Build history of the part. All positions in model axes, mm. Face numbers are marked on the shaded views. A direction names the side the tool comes from. Round coordinates to 2 decimals unless told otherwise and drop trailing zeros. Write each loop counter-clockwise with the first axis right and the second up, starting at its lowest first coordinate (ties: lowest second). Pieces come first, ordered by that corner, then holes. Notation, with made-up numbers: M 3.25,11.5 L 26.25,11.5 A34 ccw 26.25,44.5 Z; hole C 49,27 d7. An arc over 180 degrees is marked long. One line per item, written item: value. Start each with the question number.
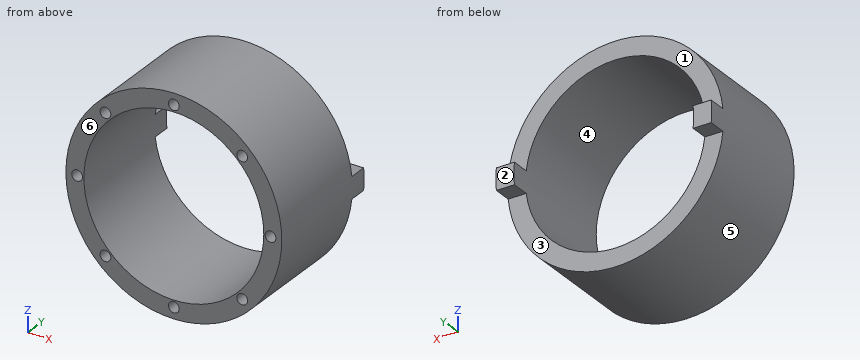
Autodesk Inventor part; units mm, degrees
ref_plane "YZ Plane" through (0, 0, 0) normal (1, 0, 0) x (0, 1, 0)
ref_plane "XZ Plane" through (0, 0, 0) normal (0, 1, 0) x (-1, 0, 0)
ref_plane "XY Plane" through (0, 0, 0) normal (0, 0, 1) x (1, 0, 0)
sketch "Sketch1" plane through (0, 0, 0) normal (0, 1, 0) x (-1, 0, 0)
  line L0 (0, 0) -> (50, 0) construction
  line L1 (0, 0) -> (50, 0) construction
  line L2 (0, 0) -> (-36, 0)
  circle A0 centre (0, 0) radius 25
  line L3 (-60, -10) -> (-60, 10)
  circle A1 centre (0, 0) radius 61
  point P0 (62.509, -33.0548)
  point P1 (12.6591, 21.558)
  point P2 (24.4148, 5.3777)
  point P3 (24.4148, -5.3777)
  point P4 (-22.9129, 10)
  point P5 (-22.9129, -10)
  point P6 (12.6591, -21.558)
  dimension "d2" = 36
  dimension "d3" = 50
  dimension "d26" = 122
extrude "Extrusion1" add sketch "Sketch1" along normal blind 5 contours A0 | A1
sketch "Sketch2" plane through (0, 5, 0) normal (0, 1, 0) x (1, 0, 0)
  circle A0 centre (0, 0) radius 20
  dimension "d6" = 40
extrude "Extrusion2" cut sketch "Sketch2" against normal up to next
sketch "Sketch3" plane through (0, 5, 0) normal (0, 1, 0) x (1, 0, 0)
  line L0 (22.1416, 4) -> (20.8701, 4)
  line L1 (22.1416, -4) -> (20.8701, -4)
  line L2 (24.6779, 4) -> (22.1416, 4)
  line L3 (24.6779, -4) -> (22.1416, -4)
  line L4 (-15.5618, -16.2506) -> (-14.5332, -15.5032)
  line L5 (-15.5618, 16.2506) -> (-14.5332, 15.5032)
  line L6 (-20.2641, -9.7784) -> (-19.2354, -9.0311)
  line L7 (-17.6137, -17.7414) -> (-15.5618, -16.2506)
  line L8 (-22.316, -11.2693) -> (-20.2641, -9.7784)
  line L9 (-20.2641, 9.7784) -> (-19.2354, 9.0311)
  line L10 (-17.6137, 17.7414) -> (-15.5618, 16.2506)
  line L11 (-22.316, 11.2693) -> (-20.2641, 9.7784)
  line L12 (-23.5374, 22.0452) -> (-13.679, 22.0452) construction
  arc A0 (-17.6137, -17.7414) -> (24.6779, -4) centre (0, 0) ccw
  arc A1 (24.6779, 4) -> (-17.6137, 17.7414) centre (0, 0) ccw
  arc A2 (-22.316, 11.2693) -> (-22.316, -11.2693) centre (0, 0) ccw
  line L13 (20.8701, 4) -> (15.8701, 4)
  line L14 (15.8701, 4) -> (15.8701, -4)
  line L15 (15.8701, -4) -> (20.8701, -4)
  line L16 (-14.5332, 15.5032) -> (-10.4881, 12.5643)
  line L17 (-10.4881, 12.5643) -> (-15.1903, 6.0922)
  line L18 (-15.1903, 6.0922) -> (-19.2354, 9.0311)
  line L19 (-19.2354, -9.0311) -> (-15.1903, -6.0922)
  line L20 (-15.1903, -6.0922) -> (-10.4881, -12.5643)
  line L21 (-10.4881, -12.5643) -> (-14.5332, -15.5032)
  circle A3 centre (-22.5, 0) radius 1.5
  circle A4 centre (0, 22.5) radius 1.5
  circle A5 centre (18.2029, 13.2252) radius 1.5
  circle A6 centre (18.2029, -13.2252) radius 1.5
  circle A7 centre (0, -22.5) radius 1.5
  circle A8 centre (0, 0) radius 4
  line L22 (0, 0) -> (8, 0)
  line L23 (8, 0) -> (8, 7.5)
  line L24 (8, 0) -> (8, -7.5)
  circle A9 centre (8, -7.5) radius 2.5
  circle A10 centre (8, 7.5) radius 2.5
  point P0 (-23.5374, -22.0452)
  point P1 (-28.2397, -15.5731)
  dimension "d9" = 36
  dimension "d10" = 5
  dimension "d11" = 5
  dimension "d12" = 3
  dimension "d13" = 3
  dimension "d14" = 3
  dimension "d15" = 3
  dimension "d16" = 3
  dimension "d17" = 8
  dimension "d18" = 8
  dimension "d19" = 7.5
  dimension "d20" = 7.5
  dimension "d21" = 5
  dimension "d22" = 5
extrude "Extrusion3" cut sketch "Sketch3" against normal up to next contours A3 | A4 | A5 | A6 | A7
sketch "Sketch5" plane through (0, 5, 0) normal (0, 1, 0) x (1, 0, 0)
  line L0 (0, 0) -> (37.5601, 0) construction
  circle A0 centre (0, 0) radius 25
  line L1 (0, 0) -> (15.7675, -27.31)
  line L2 (0, 0) -> (31.5349, 0) construction
  line L3 (0, 0) -> (19.8269, 34.3411)
  line L4 (0, 0) -> (39.6537, 0) construction
  line L5 (12.5, 21.6506) -> (15, 25.9808)
  line L6 (12.5, -21.6506) -> (15, -25.9808)
  line L7 (15, -25.9808) -> (27.9904, -18.4808)
  line L8 (27.9904, -18.4808) -> (34.9904, -30.6051)
  line L9 (34.9904, -30.6051) -> (22, -38.1051)
  line L10 (22, -38.1051) -> (15, -25.9808)
  line L11 (22, -38.1051) -> (15, -25.9808)
  line L12 (15, -25.9808) -> (2.0096, -33.4808)
  line L13 (2.0096, -33.4808) -> (9.0096, -45.6051)
  line L14 (9.0096, -45.6051) -> (22, -38.1051)
  line L15 (15, 25.9808) -> (2.0096, 33.4808)
  line L16 (2.0096, 33.4808) -> (9.0096, 45.6051)
  line L17 (9.0096, 45.6051) -> (22, 38.1051)
  line L18 (22, 38.1051) -> (15, 25.9808)
  line L19 (22, 38.1051) -> (15, 25.9808)
  line L20 (15, 25.9808) -> (27.9904, 18.4808)
  line L21 (27.9904, 18.4808) -> (34.9904, 30.6051)
  line L22 (34.9904, 30.6051) -> (22, 38.1051)
  dimension "d41" = 50
  dimension "d47" = 60
  dimension "d48" = 60
  dimension "d49" = 5
  dimension "d50" = 5
  dimension "d51" = 15
  dimension "d52" = 14
  dimension "d53" = 15
  dimension "d54" = 15
  dimension "d55" = 14
  dimension "d56" = 15
extrude "Extrusion5" cut sketch "Sketch5" against normal up to next contours L7 L8 L9 L10 L1 | L1 L10 L14 L13 L12 | L15 L16 L17 L18 L3 | L3 L18 L22 L21 L20
sketch "Sketch6" plane through (0, 0, 0) normal (0, -1, 0) x (1, 0, 0)
  circle A0 centre (0, 0) radius 25
  circle A1 centre (0, 0) radius 28.75
  circle A2 centre (0, 0) radius 30
  dimension "d57" = 50
  dimension "d58" = 57.5
extrude "Extrusion6" add sketch "Sketch6" along normal blind 30 contours A1 | A2
sketch "Sketch7" plane through (0, -30, 0) normal (0, -1, 0) x (1, 0, 0)
  circle A0 centre (26.875, 0) radius 1.5
  circle A1 centre (0, -26.875) radius 1.5
  circle A2 centre (-26.875, 0) radius 1.5
  circle A3 centre (0, 26.875) radius 1.5
  circle A4 centre (19.0035, 19.0035) radius 1.5
  circle A5 centre (19.0035, -19.0035) radius 1.5
  circle A6 centre (-19.0035, -19.0035) radius 1.5
  circle A7 centre (-19.0035, 19.0035) radius 1.5
  dimension "d62" = 3
  dimension "d63" = 3
  dimension "d64" = 3
  dimension "d65" = 3
  dimension "d67" = 3
  dimension "d68" = 3
  dimension "d69" = 3
  dimension "d70" = 3
extrude "Extrusion7" cut sketch "Sketch7" against normal blind 10
sketch "Sketch8" plane through (0, 0, 0) normal (0, -1, 0) x (1, 0, 0)
  line L0 (-37.9479, -22.6265) -> (-41.4746, -17.7724)
  line L1 (-47.9467, -22.4747) -> (-44.42, -27.3288)
  line L2 (-31.2231, -27.6292) -> (-27.6611, -32.4577)
  circle A0 centre (-42.9473, -22.5506) radius 1.5
  circle A1 centre (-26.2405, -27.6816) radius 1.5
  line L3 (-29.7189, 33.9527) -> (-36.191, 38.655)
  line L4 (-39.7177, 33.8009) -> (-33.2456, 29.0986)
  line L5 (-29.4532, 16.4547) -> (-35.9253, 21.157)
  line L6 (41.5, 10) -> (33.5, 10)
  line L7 (33.5, 4) -> (41.5, 4)
  line L8 (44, -10) -> (52, -10)
  circle A2 centre (48, -7) radius 1.5
  circle A3 centre (37.5, 7) radius 1.5
  circle A4 centre (-34.7183, 33.8768) radius 1.5
  circle A5 centre (-34.4526, 16.3788) radius 1.5
  point P0 (0, 0)
  point P1 (0, 0)
  point P2 (-32.9799, 11.6006)
  point P3 (44, -4)
  dimension "d73" = 3
  dimension "d74" = 3
  dimension "d75" = 3
  dimension "d76" = 3
  dimension "d77" = 3
extrude "Extrusion8" cut sketch "Sketch8" against normal blind 5
sketch "Sketch9" plane through (0, 5, 0) normal (0, 1, 0) x (1, 0, 0)
  line L0 (2.0096, -33.4808) -> (27.9904, -18.4808)
  line L1 (9.0096, -45.6051) -> (2.0096, -33.4808)
  line L2 (2.0096, -33.4808) -> (-0.5885, -34.9808)
  line L3 (-0.5885, -34.9808) -> (6.4115, -47.1051)
  line L4 (6.4115, -47.1051) -> (9.0096, -45.6051)
  line L5 (2.0096, 33.4808) -> (9.0096, 45.6051)
  line L6 (2.0096, 33.4808) -> (9.0096, 45.6051)
  line L7 (9.0096, 45.6051) -> (6.4115, 47.1051)
  line L8 (6.4115, 47.1051) -> (-0.5885, 34.9808)
  line L9 (-0.5885, 34.9808) -> (2.0096, 33.4808)
  point P0 (0, 0)
  dimension "d80" = 3
  dimension "d81" = 3
extrude "Extrusion9" cut sketch "Sketch9" against normal blind 10
sketch "Sketch10" plane through (0, 0, 0) normal (0, -1, 0) x (1, 0, 0)
  line L0 (6.4115, 47.1051) -> (-9.1769, 56.1051)
  line L1 (-9.1769, 56.1051) -> (-16.1769, 43.9808)
  line L2 (-16.1769, 43.9808) -> (-0.5885, 34.9808)
  line L3 (-9.1769, 56.1051) -> (-11.1769, 52.641)
  line L4 (-16.1769, 43.9808) -> (-14.1769, 47.4449)
  line L5 (-0.5885, 34.9808) -> (1.4115, 38.4449)
  line L6 (1.4115, 38.4449) -> (-2.0526, 40.4449)
  line L7 (6.4115, 47.1051) -> (4.4115, 43.641)
  line L8 (-0.5885, 34.9808) -> (6.4115, 47.1051)
  line L9 (4.4115, 43.641) -> (0.9474, 45.641)
  line L10 (27.9904, -18.4808) -> (-0.5885, -34.9808)
  line L11 (-16.1769, -43.9808) -> (-9.1769, -56.1051)
  line L12 (6.4115, -47.1051) -> (-0.5885, -34.9808)
  line L13 (-16.1769, -43.9808) -> (-14.1769, -47.4449)
  line L14 (-14.1769, -47.4449) -> (-10.7128, -45.4449)
  line L15 (-9.1769, -56.1051) -> (-11.1769, -52.641)
  line L16 (6.4115, -47.1051) -> (4.4115, -43.641)
  line L17 (-0.5885, -34.9808) -> (6.4115, -47.1051)
  line L18 (-0.5885, -34.9808) -> (1.4115, -38.4449)
  line L19 (6.4115, 47.1051) -> (3.8135, 48.6051)
  line L20 (3.8135, 48.6051) -> (-3.1865, 36.4808)
  line L21 (3.8135, 48.6051) -> (-2.6817, 52.3551)
  line L22 (1.8135, 45.141) -> (-2.0836, 47.391)
  line L23 (-2.0836, 47.391) -> (-5.0836, 42.1949)
  line L24 (-0.5885, -34.9808) -> (1.4115, -38.4449)
  line L25 (6.4115, -47.1051) -> (4.4115, -43.641)
  circle A0 centre (-5.5836, -41.3288) radius 1.5
  circle A1 centre (-1.5836, -48.257) radius 1.5
  line L26 (-2.0836, 47.391) -> (-1.5836, 48.257)
  line L27 (-5.0836, 42.1949) -> (-5.5836, 41.3288)
  circle A2 centre (-1.5836, 48.257) radius 1.5
  circle A3 centre (-5.5836, 41.3288) radius 1.5
  point P0 (0, 0)
  dimension "d85" = 14
  dimension "d86" = 4
  dimension "d88" = 4
  dimension "d92" = 4
  dimension "d93" = 4
  dimension "d94" = 4
  dimension "d95" = 4
  dimension "d98" = 18
  dimension "d99" = 4
  dimension "d101" = 4
  dimension "d103" = 4
  dimension "d129" = 3
  dimension "d130" = 7.5
  dimension "d137" = 4.5
  dimension "d140" = 4
  dimension "d146" = 3
  dimension "d148" = 1
  dimension "d149" = 1
  dimension "d150" = 3
  dimension "d151" = 3
extrude "Extrusion13" cut sketch "Sketch10" against normal blind 10 contours A2 L23 L22 | L22 L23 A2 | A0 | A1 | A3
sketch "Sketch11" plane through (0, 5, 0) normal (0, 1, 0) x (1, 0, 0)
  circle A0 centre (0, 0) radius 61
extrude "Extrusion14" cut sketch "Sketch11" against normal blind 5
sketch "Sketch12" plane through (0, 0, 0) normal (0, 1, 0) x (1, 0, 0)
  circle A0 centre (0, 0) radius 30
  circle A1 centre (0, 0) radius 30
  circle A2 centre (0, 0) radius 25
  circle A3 centre (0, 0) radius 25
  line L0 (-25, -3) -> (-29.8496, -3)
  line L1 (-24.8193, -3) -> (-25, -3)
  line L2 (-25, 3) -> (-24.8193, 3)
  line L3 (-29.8496, 3) -> (-24.8193, 3)
  line L4 (24.8193, -3) -> (29.8496, -3)
  line L5 (24.8193, 3) -> (29.8496, 3)
extrude "Extrusion15" add sketch "Sketch12" along normal blind 5 contours A0 L4 A2 L5 | L3 L2 A2 L1 L0 A0
properties part number "upperBase1"
Item 1: Drill centre lines: line 1 (Z direction, x = 0, y = -25) (3 decimals); line 2 (X direction, y = -13, z = -18.5); line 3 (Z direction, x = 1, y = -3.5). Where is each one in solid material? Low to high.
Item 2: Cut at C-C, the plane y = -21.5. Count the separate pieces of the cut face and the enclosed holes in it, plus the area to 3 significant figures.
Item 3: Drop flat-ended pins along their axis: pin 1 (10 mm diameter, centred on x = 12.5, y = -19, fed in from -Z); pin 2 (6 mm diameter, centred on y = -9, z = 0.5, fed in from +X); pin 3 (2 mm diameter, centred on x = 5.5, y = -3, fed in from -Z); pin 4 (2.5 mm diameter, centred on x = 0, z = 26.875, fed in from -Y). Give the stop position or say it passes through.
Item 4: Cut at B-B, the plane x = 0. Write the cut outline in (y, z) (3 decimals).
Item 5: Two-plate mould, pull along Z, no slides. Class the marked faces 4, 5 and 6: pulls with the +Z half, pulls with the -Z half, needs draft (parallel to the pull), parting line crosses it, or undercut.
Item 6: Cut at A-A, the plane z = 0. Write the cut outline in (x, y) (3 decimals), plus the area to 3 significant figures.
Item 7: Cut at D-D, the plane y = -8. Write the cut outline in (x, z), plus the area to 3 significant figures.
Item 8: Which spindle directions (+Z, -Z, +X, -X, +Y, -Y) get a long thin tool onto all of the face, cutting with end or side? Do the marked faces 1, 2 and 3. Say none if no direction does.
Computed values:
1. line 1: z = -30 to -28.375, -25.375 to -25, 25 to 25.375, 28.375 to 30
1. line 2: x = -23.62 to -16.82, 16.82 to 23.62
1. line 3: z = -29.98 to -24.98, 24.98 to 29.98
2. separate pieces: 1
2. enclosed holes: 9
2. area: 807 mm2
3. pin 1: stops at z = -29.05
3. pin 2: stops at x = 30
3. pin 3: stops at z = -29.66
3. pin 4: stops at y = -20
4. outline: M -30,-30 L 0,-30 L 0,-25 L -30,-25 L -30,-25.375 L -20,-25.375 L -20,-28.375 L -30,-28.375 Z; M -30,25 L 0,25 L 0,30 L -30,30 L -30,28.375 L -20,28.375 L -20,25.375 L -30,25.375 Z
5. face 4: undercut
5. face 5: parting line crosses it
5. face 6: needs draft
6. outline: M -30,-30 L -28.375,-30 L -28.375,-20 L -25.375,-20 L -25.375,-30 L -25,-30 L -25,5 L -30,5 Z; M 25,-30 L 25.375,-30 L 25.375,-20 L 28.375,-20 L 28.375,-30 L 30,-30 L 30,5 L 25,5 Z
6. area: 290 mm2
7. outline: C 0,0 d60; hole C 0,0 d50
7. area: 864 mm2
8. face 1: +Z, +X, -X, +Y
8. face 2: +Z, -Z, +X, -X, +Y
8. face 3: -Z, +X, -X, +Y
